```python
from build123d import *

# Parameters (mm, degrees)
SKETCH_W        = 508
SKETCH_H        = 31.75
PAD_DEPTH       = 25.4
SKETCH001_W     = 25.4
SKETCH001_H     = 6.35
POCKET_DEPTH    = 25.401
SKETCH002_W     = 25.4
SKETCH002_H     = 6.35
POCKET001_DEPTH = 25.401
SKETCH003_R     = 3.175
POCKET002_DEPTH = 31.751


with BuildPart() as part:
    # Sketch → Pad (new body)
    with BuildSketch(Plane.XZ):
        Rectangle(SKETCH_W, SKETCH_H)
    extrude(amount=PAD_DEPTH)

    # Sketch001 (on Face6 of Pad) → Pocket (cut, through all)
    with BuildSketch(Plane.XZ.offset(25.4)):
        with Locations((-241.3, 12.7)):
            Rectangle(SKETCH001_W, SKETCH001_H)
        with Locations((-241.3, 0)):
            Rectangle(SKETCH001_W, SKETCH001_H)
        with Locations((-241.3, -12.7)):
            Rectangle(SKETCH001_W, SKETCH001_H)
    extrude(amount=-POCKET_DEPTH, mode=Mode.SUBTRACT)

    # Sketch002 (on Face6 of Pad) → Pocket001 (cut, through all)
    with BuildSketch(Plane.XZ.offset(25.4)):
        with Locations((241.3, 6.35)):
            Rectangle(SKETCH002_W, SKETCH002_H)
        with Locations((241.3, -6.35)):
            Rectangle(SKETCH002_W, SKETCH002_H)
    extrude(amount=-POCKET001_DEPTH, mode=Mode.SUBTRACT)

    # Sketch003 (on Face11 of Pocket001) → Pocket002 (cut, through all)
    with BuildSketch(Plane(origin=(0, 0, -15.875), x_dir=(1, 0, 0), z_dir=(0, 0, -1))):
        with Locations((-241.3, 12.7)):
            Circle(SKETCH003_R)
        with Locations((241.3, 12.7)):
            Circle(SKETCH003_R)
    extrude(amount=-POCKET002_DEPTH, mode=Mode.SUBTRACT)


solid = part.part
```
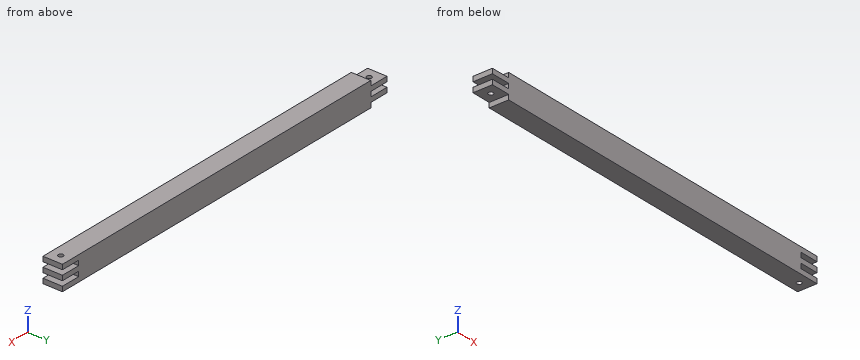
The model under review builds one solid part; all positions refer to its coordinate system, in mm. Coordinates: 2 decimals unless noted, no trailing zeros. Write each loop counter-clockwise with the first axis right and the second up, starting at its lowest first coordinate (ties: lowest second). Pieces come first, ordered by that corner, then holes. Notation, with made-up numbers: (15, -13) - (48, -13) arc R21 ccw to (48, 19) - close; hole circle Ø3 at (-36.5, 5). An arc over 180 degrees is marked (long way). Answer in a Markdown table with one row per item. Add a question column.
Q1. Clearance check with flat-ended pins moving along their axes: pin 1 (7.5 mm diameter, centred on x = -236.5, y = -13.5, fed in from -Z) (3 decimals); pin 2 (7.5 mm diameter, centred on x = -241.3, y = -12.7, fed in from +Z) (3 decimals); pin 3 (1.9 mm diameter, centred on y = -9, z = -14, fed in from -X). State where each tip first meets the part, or that it passes through.
Q2. To check wall thickness, follow line 1 along X through (y, z) = (-12.7, 1.75) (3 decimals); line 2 along Y through (x, z) = (-241.3, -4.5) (3 decimals); line 3 along X through (y, z) = (-12.7, 7.25) (3 decimals). State the ranges of each line that lie inside material, in increasing order. Write a range as from..to.
Q3. Consider section A-A on y = -21. Give the boundary of the cut face in (x, z) (3 decimals).
Answers below:
| question | item | result |
|---|---|---|
| 1 | pin 1 | z = -9.525 |
| 1 | pin 2 | z = 9.525 |
| 1 | pin 3 | x = -228.6 |
| 2 | line 1 | -228.6..238.125, 244.475..254 |
| 2 | line 2 | -25.4..-15.875, -9.525..0 |
| 2 | line 3 | -254..-244.475, -238.125..228.6 |
| 3 | outline | (-254, -9.525) - (-228.6, -9.525) - (-228.6, -15.875) - (254, -15.875) - (254, -9.525) - (228.6, -9.525) - (228.6, -3.175) - (254, -3.175) - (254, 3.175) - (228.6, 3.175) - (228.6, 9.525) - (254, 9.525) - (254, 15.875) - (-228.6, 15.875) - (-228.6, 9.525) - (-254, 9.525) - (-254, 3.175) - (-228.6, 3.175) - (-228.6, -3.175) - (-254, -3.175) - close |
